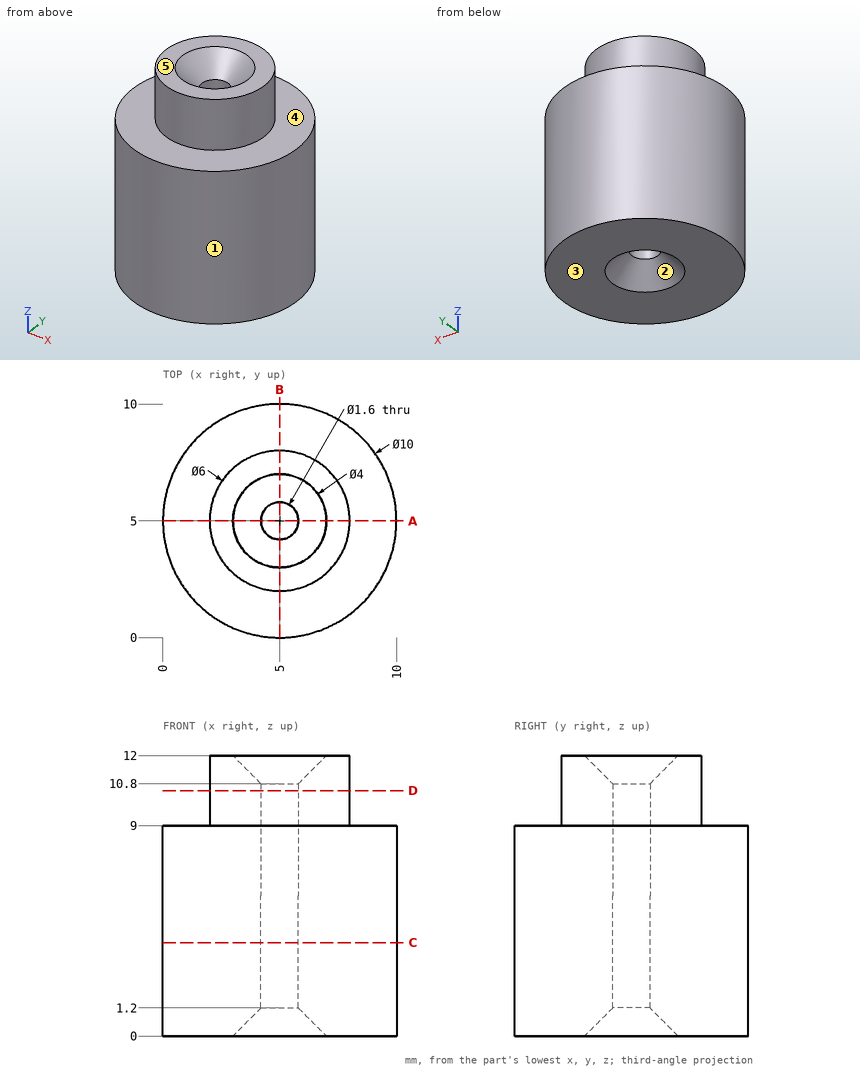
Design review of the part shown in the three views and the two pictorial views. Dimensions are in mm from the part's minimum x, y and z. A direction names the side the tool comes from. Give positions to 0.01 mm unless a question says otherwise; leave off trailing zeros. Write each loop counter-clockwise with the first axis right and the second up, starting at its lowest first coordinate (ties: lowest second). Pieces come first, ordered by that corner, then holes. Notation, with made-up numbers: (79.5, 85) - (89.5, 85) arc R24 cw to (89.5, 121) - close; hole circle Ø8 at (71, 7.25). An arc over 180 degrees is marked (long way). Return JSON: item names as keys, results as strings. Group by question number.
(1) We need section C-C, the plane z = 4. Give the boundary of the cut face in (x, y).
(2) To check wall thickness, follow probe 1 along Y at (x, z) = (5, 4.2); probe 2 along Y at (x, z) = (5, 9.6); probe 3 along Z at (x, y) = (8.25, 2). State the ranges of each line that lie inside material, in increasing order.
(3) Mouldability with a two-part tool opening along X and no side actions: class the marked faces 1, 2 and 3 as +X half, -X half, draft (parallel to the pull), parting line (faces both ways), or undercut.
(4) We need section A-A, the plane y = 5. Give the boundary of the cut face in (x, z).
(5) Machinability: for the marked faces 4 and 5, which of the approach directions +Z, -Z, +X, -X, +Y, -Y give a long, thin tool a straight path to every point of the face, cutting with its end or side? Answer none if there is none.
(6) We need section D-D, the plane z = 10.5. Give the boundary of the cut face in (x, y).
(7) Insertion check: pin 1 (2 mm diameter, centred on y = 9, z = 2.5, fed in from -X); pin 2 (1 mm diameter, centred on y = 4.5, z = 2, fed in from +X); pin 3 (3 mm diameter, centred on x = 8, z = 11, fed in from +Y); pin 4 (1.5 mm diameter, centred on x = 6, z = 3.5, fed in from +Y). Each pin has a flat end and moves straight along its axis. Give the tip position at first contact, or say it passes through.
Reported:
{
 "1": {"outline": "circle Ø10 at (5, 5); hole circle Ø1.6 at (5, 5)"},
 "2": {"probe 1": "y = 0 to 4.2, 5.8 to 10", "probe 2": "y = 2 to 4.2, 5.8 to 8", "probe 3": "z = 0 to 9"},
 "3": {"face 1": "parting line", "face 2": "undercut", "face 3": "draft"},
 "4": {"outline": "(0, 0) - (3, 0) - (4.2, 1.2) - (4.2, 10.8) - (3, 12) - (2, 12) - (2, 9) - (0, 9) - close; (5.8, 1.2) - (7, 0) - (10, 0) - (10, 9) - (8, 9) - (8, 12) - (7, 12) - (5.8, 10.8) - close"},
 "5": {"face 4": "+Z", "face 5": "+Z, +X, -X, +Y, -Y"},
 "6": {"outline": "circle Ø6 at (5, 5); hole circle Ø1.6 at (5, 5)"},
 "7": {"pin 1": "stops at x = 1", "pin 2": "stops at x = 10", "pin 3": "stops at y = 7.6", "pin 4": "stops at y = 9.99"}
}
